The model under review builds one solid part; all positions refer to its coordinate system, in mm. A direction names the side the tool comes from. Give positions to 0.01 mm unless a question says otherwise; leave off trailing zeros. Order: outer loops, then holes, each group sorted by start corner. A loop starts at its lowest first (then second) coordinate and runs counter-clockwise, first axis right, second up. Notation, with made-up numbers: (74.25, 50) - (87.25, 50) arc R11 ccw to (87.25, 62) - close; hole circle Ø9 at (-36.75, 4.25). An arc over 180 degrees is marked (long way). Use CSV: the item, a comma, the result in double quotes. Start each with the question number.
1. For pin 1 (6 mm diameter, centred on x = 32.5, y = 16.5, fed in from +Z); pin 2 (12 mm diameter, centred on x = -3.5, y = 108, fed in from -Z); pin 3 (4 mm diameter, centred on x = 9, z = -51.5, fed in from +Y), all flat-tipped, find the tip position at first contact; note any pin that passes through.
2. Draft analysis for pull direction Z (two halves, no side actions). For faces 1 (the flat face through (25.45, 74, 1)), 2 (the cylindrical face through (56.03, 132.23, -18.02)), 3 (the cylindrical face through (47.635, 127.716, 11.706)), 4 (the flat face through (70.45, 21, 9)), state which applies: released by +Z, released by -Z, zero draft, split by the parting line, or undercut.
3. To check wall thickness, follow line 1 (Z direction, x = 42, y = 75); line 2 (Y direction, x = 49, z = 0); line 3 (Z direction, x = 50, y = 70). State the ranges of each line that lie inside material, in increasing order. Write a range as [from, to].
4. Take a section at B-B, the plane y = 46. State the section outline as (x, z) points.
5. Take a section at A-A, the plane x = 53.5. State the section outline as (y, z) points, then the cut area to 3 significant figures.
6. Machinability: for faces 5 (the flat face through (-1, 0, 1)), 6 (the cylindrical face through (-64.937, 25.384, -2.858)), which of the approach directions +Z, -Z, +X, -X, +Y, -Y give a long, thin tool a straight path to every point of the face, cutting with its end or side? Answer none if there is none.
Autodesk Inventor part; units mm, degrees
ref_plane "YZ Plane" through (0, 0, 0) normal (1, 0, 0) x (0, 1, 0)
ref_plane "XZ Plane" through (0, 0, 0) normal (0, 1, 0) x (-1, 0, 0)
ref_plane "XY Plane" through (0, 0, 0) normal (0, 0, 1) x (1, 0, 0)
sketch "Sketch1" plane through (0, 0, 0) normal (0, 0, 1) x (1, 0, 0)
  line L0 (0, 0) -> (65, 0)
  line L1 (0, 126.1861) -> (0, 150)
  line L2 (0, 18.2402) -> (0, 0)
  line L3 (0, 126.1861) -> (0, 18.2402)
  line L4 (65, 0) -> (65, 50.0668)
  line L5 (0, 150) -> (62.6016, 156.9829) construction
  line L6 (62.6016, 156.9829) -> (70.4299, 73.1619) construction
  spline S0 degree 2 poles (0, 150) (62.6016, 156.9829) (70.4299, 73.1619) knots 1 1 1 2 2 2
  line L7 (65, 50.0668) -> (70.4299, 73.1619) construction
  spline S1 degree 1 poles (65, 50.0668) (70.4299, 73.1619) knots 1 1 2 2
  point P0 (84.7515, 38.5438)
  dimension "d1" = 65
  dimension "d2" = 150
revolve "Revolution1" add sketch "Sketch1" angle 360 about axis through (0, 126.1861, 0) along (0, -1, 0)
sketch "Sketch2" plane through (0, 0, 0) normal (1, 0, 0) x (0, 1, 0)
  line L0 (0, 75) -> (0, -75)
  circle A0 centre (75, 0) radius 60
  point P0 (0, 0)
  point P1 (150, 0)
  dimension "d4" = 120
  dimension "d25" = 75
extrude "Extrusion1" add sketch "Sketch2" along normal blind 70.45
hole "Hole1" at (70.45, 75, 0) direction (-1, 0, 0) diameter 108 depth 45
properties part number "tete2"
Determined:
1,pin 1,"stops at z = 57.92"
1,pin 2,"stops at z = -65.33"
1,pin 3,"stops at y = 132.73"
2,face 1,"undercut"
2,face 2,"split by the parting line"
2,face 3,"undercut"
2,face 4,"zero draft"
3,line 1,"z = [-60, -54], [54, 60]"
3,line 2,"y = [0, 21], [129, 135]"
3,line 3,"z = [-59.79, -53.77], [53.77, 59.79]"
4,outline,"(25.45, -45.55) - (25.45, 45.55) - (70.45, 45.55) - (70.45, 52.53) - (38.29, 52.53) arc R65 ccw (long way) to (38.29, -52.53) - (70.45, -52.53) - (70.45, -45.55) - close"
5,outline,"(0, -36.92) - (27.7, -36.92) arc R60 ccw (long way) to (27.7, 36.92) - (0, 36.92) - close; hole circle Ø108 at (75, 0)"
5,area,"3,550 mm²"
6,face 5,"+Z, -Z, +X, -X, -Y"
6,face 6,"-Y"
